Could you check a few things on this model? Use its own coordinates, in mm. A direction names the side the tool comes from. Coordinates: 2 decimals unless noted, no trailing zeros. Write each loop counter-clockwise with the first axis right and the second up, starting at its lowest first coordinate (ties: lowest second). Pieces come first, ordered by that corner, then holes. Notation, with made-up numbers: M 29,-8 L 68,-8 A25 ccw 68,9 Z; hole C -24.75,75 d2. An arc over 180 degrees is marked long. Write item = value, one per line.
```python
from build123d import *

# Parameters (mm, degrees)
EXTRUDE_1_DEPTH = 10
EXTRUDE_2_DEPTH = 13


with BuildPart() as part:
    # Эскиз1 → Повернуть1 (revolve)
    with BuildSketch(Plane.XY, mode=Mode.PRIVATE) as revolve_1_sk:
        Polygon((0, 0), (-50, 0), (-50, 18), (-42, 26), (-20, 26), (-20, 29), (-8, 29), (-8, 39), (-8, 187), (-6, 189), (0, 189), align=None)
    revolve(revolve_1_sk.sketch.rotate(Axis((0, 0, 0), (0, 1, 0)), 180), axis=Axis((0, 0, 0), (0, 1, 0)))  # turned: the seam where the file's is

    # Эскиз2 → Бобышка-Вытянуть1 (add)
    with BuildSketch(Plane(origin=(0, 29, 0), x_dir=(1, 0, 0), z_dir=(0, 1, 0))):
        Polygon((0, 13.856406461), (-12, 6.92820323), (-12, -6.92820323), (0, -13.856406461), (12, -6.92820323), (12, 6.92820323), align=None)
    extrude(amount=EXTRUDE_1_DEPTH)

    # Эскиз3 → Бобышка-Вытянуть2 (add)
    with BuildSketch(Plane(origin=(0, 113, 0), x_dir=(1, 0, 0), z_dir=(0, 1, 0))):
        Polygon((12, 6.92820323), (0, 13.856406461), (-12, 6.92820323), (-12, -6.92820323), (0, -13.856406461), (12, -6.92820323), align=None)
    extrude(amount=EXTRUDE_2_DEPTH)

    # Эскиз4 → Вырез-Повернуть2 (revolve, cut)
    with BuildSketch(Plane.XY, mode=Mode.PRIVATE) as cut_revolve_2_sk:
        Polygon((-23.258330249, 126), (-12, 126), (-23.258330249, 119.5), align=None)
        Polygon((-23.258330249, 113), (-23.258330249, 119.5), (-12, 113), align=None)
        Polygon((-20.660254038, 39), (-20.660254038, 34), (-12, 39), align=None)
        Polygon((-20.660254038, 34), (-20.660254038, 29), (-12, 29), align=None)
    revolve(cut_revolve_2_sk.sketch.rotate(Axis((0, 189, 0), (0, -1, 0)), 180), axis=Axis((0, 189, 0), (0, -1, 0)), mode=Mode.SUBTRACT)  # turned: the seam where the file's is


solid = part.part
```
Item 1: Imagine slicing it at A-A (y = 116.5). Write out the boundary of the cut face in (x, z).
Numbers:
outline = M -12,-6.93 L 0,-13.86 L 12,-6.93 L 12,6.93 L 0,13.86 L -12,6.93 Z
Item 2: I'm going to push flat-ended pins straight in: P1, Ø6, axis at x = -6.5, y = 57, coming from the -Z side; P2, Ø6.5, axis at y = 119.5, z = -3, coming from the -X side; P3, Ø5, axis at x = 9, y = 167.5, coming from the +Z side. Where does each tip first touch, or does it pass through?
Numbers:
P1 = -7.19
P2 = -12
P3 = 4.66
Item 3: For faces 1 (the face through (5.92, 33.93, 10.44)), 2 (the face through (12, 34, 0)), 3 (the face through (6.084, 119.409, -10.344)), 4 (the face through (-6.084, 33.93, 10.344)), which set-ups out of +Z, -Z, +X, -X, +Y, -Y let a thin tool reach every point of the face, with its end or its side?
Numbers:
face_1 = +Z, +X, +Y
face_2 = +Z, -Z, +X, +Y
face_3 = -Z, +X, +Y
face_4 = +Z, -X, +Y
Item 4: If I drill on line 1 along Y through (x, z) = (-34.5, -16); line 2 along Y through (x, z) = (-13, -5.5); line 3 along X through (y, z) = (100, 6), over which ranges is the centre line in solid material (lowest first)?
Numbers:
line_1 = 0 to 26
line_2 = 0 to 29
line_3 = -5.29 to 5.29
